Build history of the part. All positions in model axes, mm. Give positions to 0.01 mm unless a question says otherwise; leave off trailing zeros. Write each loop counter-clockwise with the first axis right and the second up, starting at its lowest first coordinate (ties: lowest second). Pieces come first, ordered by that corner, then holes. Notation, with made-up numbers: M 63.5,25 L 90.5,25 A13 ccw 90.5,42 Z; hole C -0.5,0.25 d3. An arc over 180 degrees is marked long. Return JSON: item names as keys, results as strings. Group by question number.
Q1. Band-saw the part on C-C, the plane x = -35.7. Give the cut face in (y, z), then the cut area to 3 significant figures.
Q2. Band-saw the part on A-A, the plane y = 0. Give the cut face in (x, z), then the cut area to 3 significant figures.
Q3. Wall check: probe 1 along Y at (x, z) = (-35.5, 2.75); probe 2 along X at (y, z) = (29.5, 1); probe 3 along Y at (x, z) = (-35.7, 1.5). Give the ranges that are in metal, low to high.
Q4. Flat gauge pins, fed straight in: pin 1 Ø3.5 at (x, y) = (-25.35, 15.47) entering from -Z; pin 2 Ø7 at (x, y) = (-25.5, 16.5) entering from +Z; pin 3 Ø0.8 at (x, z) = (-36, 1.5) entering from +Y; pin 4 Ø1.2 at (y, z) = (-35.5, 1) entering from -X. Where does each tip first touch, or does it go through?
from build123d import *

# Parameters (mm, degrees)
SKETCH1_R           = 1.5
SKETCH1_R_2         = 25
BOSS_EXTRUDE1_DEPTH = 2.5
SKETCH2_R           = 3.25
CUT_EXTRUDE1_DEPTH  = 0.5
SKETCH4_R           = 4.5
SKETCH4_R_2         = 1.5
BOSS_EXTRUDE2_DEPTH = 2


with BuildPart() as part:
    # Sketch1 → Boss-Extrude1 (new body)
    with BuildSketch(Plane.XY):
        with BuildLine():
            Line((34.373350084, -40), (37.026649916, -40))
            ThreePointArc((37.026649916, -40), (38.881980515, -38.881980515), (40, -37.026649916))
            Line((40, -37.026649916), (40, -34.373350084))
            ThreePointArc((40, -34.373350084), (39.554292544, -33.377408993), (38.881980515, -32.518019485))
            Line((38.881980515, -32.518019485), (27.930717857, -21.566756826))
            ThreePointArc((27.930717857, -21.566756826), (27.826741101, -21.466071831), (27.719580149, -21.368782754))
            ThreePointArc((27.719580149, -21.368782754), (28.839517017, -19.831345346), (29.874277905, -18.235337114))
            ThreePointArc((29.874277905, -18.235337114), (30.48642799, -14.163770708), (28, -10.881994271))
            Line((28, -10.881994271), (28, 21.636038969))
            Line((28, 21.636038969), (38.881980515, 32.518019485))
            ThreePointArc((38.881980515, 32.518019485), (39.554292544, 33.377408993), (40, 34.373350084))
            Line((40, 34.373350084), (40, 37.026649916))
            ThreePointArc((40, 37.026649916), (38.881980515, 38.881980515), (37.026649916, 40))
            Line((37.026649916, 40), (34.373350084, 40))
            ThreePointArc((34.373350084, 40), (33.377408993, 39.554292544), (32.518019485, 38.881980515))
            Line((32.518019485, 38.881980515), (21.566756826, 27.930717857))
            ThreePointArc((21.566756826, 27.930717857), (21.466071831, 27.826741101), (21.368782754, 27.719580149))
            ThreePointArc((21.368782754, 27.719580149), (19.831345346, 28.839517017), (18.235337114, 29.874277905))
            ThreePointArc((18.235337114, 29.874277905), (14.163770708, 30.48642799), (10.881994271, 28))
            Line((10.881994271, 28), (-21.636038969, 28))
            Line((-21.636038969, 28), (-32.518019485, 38.881980515))
            ThreePointArc((-32.518019485, 38.881980515), (-33.377408993, 39.554292544), (-34.373350084, 40))
            Line((-34.373350084, 40), (-37.026649916, 40))
            ThreePointArc((-37.026649916, 40), (-38.881980515, 38.881980515), (-40, 37.026649916))
            Line((-40, 37.026649916), (-40, 34.373350084))
            ThreePointArc((-40, 34.373350084), (-39.554292544, 33.377408993), (-38.881980515, 32.518019485))
            Line((-38.881980515, 32.518019485), (-27.930717857, 21.566756826))
            ThreePointArc((-27.930717857, 21.566756826), (-27.826741101, 21.466071831), (-27.719580149, 21.368782754))
            ThreePointArc((-27.719580149, 21.368782754), (-28.839517017, 19.831345346), (-29.874277905, 18.235337114))
            ThreePointArc((-29.874277905, 18.235337114), (-30.48642799, 14.163770708), (-28, 10.881994271))
            Line((-28, 10.881994271), (-28, -21.636038969))
            Line((-28, -21.636038969), (-38.881980515, -32.518019485))
            ThreePointArc((-38.881980515, -32.518019485), (-39.554292544, -33.377408993), (-40, -34.373350084))
            Line((-40, -34.373350084), (-40, -37.026649916))
            ThreePointArc((-40, -37.026649916), (-38.881980515, -38.881980515), (-37.026649916, -40))
            Line((-37.026649916, -40), (-34.373350084, -40))
            ThreePointArc((-34.373350084, -40), (-33.377408993, -39.554292544), (-32.518019485, -38.881980515))
            Line((-32.518019485, -38.881980515), (-21.566756826, -27.930717857))
            ThreePointArc((-21.566756826, -27.930717857), (-21.466071831, -27.826741101), (-21.368782754, -27.719580149))
            ThreePointArc((-21.368782754, -27.719580149), (-19.831345346, -28.839517017), (-18.235337114, -29.874277905))
            ThreePointArc((-18.235337114, -29.874277905), (-14.163770708, -30.48642799), (-10.881994271, -28))
            Line((-10.881994271, -28), (21.636038969, -28))
            Line((21.636038969, -28), (32.518019485, -38.881980515))
            ThreePointArc((32.518019485, -38.881980515), (33.377408993, -39.554292544), (34.373350084, -40))
        make_face()
        with Locations((-35.7, -35.7)):
            Circle(SKETCH1_R, mode=Mode.SUBTRACT)
        with Locations((-15.473196637, -25.349165387)):
            Circle(SKETCH1_R, mode=Mode.SUBTRACT)
        with Locations((35.7, -35.7)):
            Circle(SKETCH1_R, mode=Mode.SUBTRACT)
        Circle(SKETCH1_R_2, mode=Mode.SUBTRACT)
        with Locations((25.349165387, -15.473196637)):
            Circle(SKETCH1_R, mode=Mode.SUBTRACT)
        with Locations((-25.349165387, 15.473196637)):
            Circle(SKETCH1_R, mode=Mode.SUBTRACT)
        with Locations((-35.7, 35.7)):
            Circle(SKETCH1_R, mode=Mode.SUBTRACT)
        with Locations((15.473196637, 25.349165387)):
            Circle(SKETCH1_R, mode=Mode.SUBTRACT)
        with Locations((35.7, 35.7)):
            Circle(SKETCH1_R, mode=Mode.SUBTRACT)
    extrude(amount=BOSS_EXTRUDE1_DEPTH)

    # Sketch2 → Cut-Extrude1 (cut)
    with BuildSketch(Plane.XY.offset(2.5)):
        with Locations((-15.473196637, -25.349165387)):
            Circle(SKETCH2_R)
        with Locations((25.349165387, -15.473196637)):
            Circle(SKETCH2_R)
        with Locations((15.473196637, 25.349165387)):
            Circle(SKETCH2_R)
        with Locations((-25.349165387, 15.473196637)):
            Circle(SKETCH2_R)
    extrude(amount=-CUT_EXTRUDE1_DEPTH, mode=Mode.SUBTRACT)

    # Sketch4 → Boss-Extrude2 (add)
    with BuildSketch(Plane.XY.offset(2.5)):
        with Locations((-35.7, 35.7)):
            Circle(SKETCH4_R)
        with Locations((-35.7, 35.7)):
            Circle(SKETCH4_R_2, mode=Mode.SUBTRACT)
        with Locations((35.7, 35.7)):
            Circle(SKETCH4_R)
        with Locations((35.7, 35.7)):
            Circle(SKETCH4_R_2, mode=Mode.SUBTRACT)
        with Locations((35.7, -35.7)):
            Circle(SKETCH4_R)
        with Locations((35.7, -35.7)):
            Circle(SKETCH4_R_2, mode=Mode.SUBTRACT)
        with Locations((-35.7, -35.7)):
            Circle(SKETCH4_R)
        with Locations((-35.7, -35.7)):
            Circle(SKETCH4_R_2, mode=Mode.SUBTRACT)
    extrude(amount=BOSS_EXTRUDE2_DEPTH)


solid = part.part
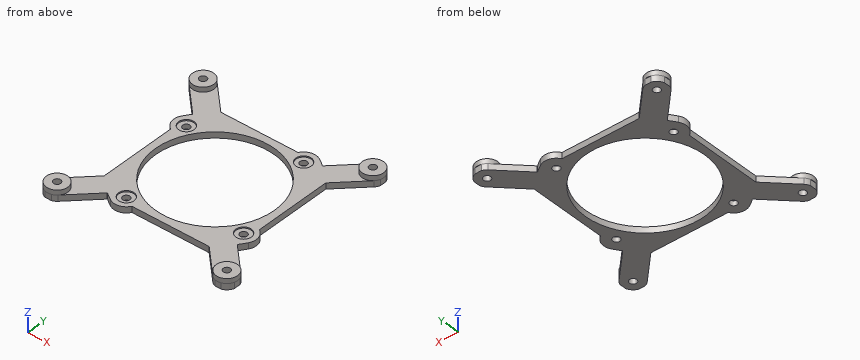
From the geometry:
{
 "1": {"outline": "M -40.2,2.5 L -40,2.5 L -40,0 L -37.2,0 L -37.2,4.5 L -40.2,4.5 Z; M -34.2,0 L -29.34,0 L -29.34,2.5 L -31.2,2.5 L -31.2,4.5 L -34.2,4.5 Z; M 29.34,0 L 34.2,0 L 34.2,4.5 L 31.2,4.5 L 31.2,2.5 L 29.34,2.5 Z; M 37.2,0 L 40,0 L 40,2.5 L 40.2,2.5 L 40.2,4.5 L 37.2,4.5 Z", "area": "62.3 mm^2"},
 "2": {"outline": "M -28,0 L -25,0 L -25,2.5 L -28,2.5 Z; M 25,0 L 28,0 L 28,2.5 L 25,2.5 Z", "area": "15.0 mm^2"},
 "3": {"probe 1": "y = -40.2 to -37.19, -34.21 to -31.2, 31.2 to 34.21, 37.19 to 40.2", "probe 2": "x = -35.86 to -23.14, 12.18 to 18.83, 23.14 to 35.86", "probe 3": "y = -40 to -37.2, -34.2 to -29.34, 29.34 to 34.2, 37.2 to 40"},
 "4": {"pin 1": "stops at z = 0", "pin 2": "stops at z = 2.5", "pin 3": "stops at y = 40", "pin 4": "stops at x = -40"}
}
